Build history of the part. All positions in model axes, mm. A direction names the side the tool comes from. Give positions to 0.01 mm unless a question says otherwise; leave off trailing zeros. Loops run counter-clockwise (first coordinate to the right, second up) from the corner with the lowest first, then second, coordinate; pieces in that order, holes last. Notation, with made-up numbers: M 50.25,62.5 L 90.25,62.5 A18 cw 90.25,91.5 Z; hole C -35.5,85.25 d5. An arc over 180 degrees is marked long. Answer in a Markdown table with one row per item. Add a question column.
```python
from build123d import *

# Parameters (mm, degrees)
F1_DEPTH = 7.62
F2_DEPTH = 3.81


with BuildPart() as f1:
    # F0 (on Front) → F1 (new body)
    with BuildSketch(Plane.XZ):
        Polygon((0, 52.186977), (-15.490659, 28.424604), (-15.490659, -28.424604), (0, -52.487765), (15.490659, -28.424604), (15.490659, 28.424604), align=None)
        Polygon((-6.466974, -17.596183), (-6.466974, 17.596183), (0, 28.424604), (6.466974, 17.596183), (6.466974, -17.596183), (0, -28.424604), align=None, mode=Mode.SUBTRACT)
    extrude(amount=F1_DEPTH)

    # F0 (on Front) → F2 (join)
    with BuildSketch(Plane.XZ):
        Polygon((0, 28.424604), (-6.466974, 17.596183), (-6.466974, -17.596183), (0, -28.424604), (6.466974, -17.596183), (6.466974, 17.596183), align=None)
    extrude(amount=F2_DEPTH)


solid = f1.part
```
(1) Slice it at B-B, the plane z = -1.5. Give the cut face in (x, y), then the cut area to 3 significant figures.
(2) Slice it at C-C, the plane y = -2.5. Give the cut face in (x, z), then the cut area to 3 significant figures.
(3) Tool access for faces 5 (the flat face through (0, -3.81, 0)), 6 (the flat face through (-7.64, -3.76, 40.47)): list every direction of +Z, -Z, +X, -X, +Y, -Y with a clear straight run to the whole face (end or side of a thin tool).
(4) Slice it at A-A, the plane y = -6.5. Give the cut face in (x, z), then the cut area to 3 significant figures.
(5) Pin check, flat tips, straight feed: pin 1 (6.5 mm diameter, centred on x = 2.5, z = -7, fed in from -Y); pin 2 (3 mm diameter, centred on x = 0.5, y = -5, fed in from -Z). Stop position of each tip, or through.
(6) Wall check: line 1 (X direction, y = -4.5, z = -7); line 2 (Z direction, x = 4, y = -6.5); line 3 (Z direction, x = -3, y = -5.25). Give the ranges that are in metal, low to high.
(7) Pull direction X, two halves, no side cores. Call faces 1 (the flat face through (-15.491, -4, 0)), 2 (the flat face through (7.854, -3.757, 40.139)), 3 (the flat face through (3.188, -5.688, 23.086)), 4 (the flat face through (-3.3, -5.7, 22.9)): +X half, -X half, draft (parallel to the pull), parting line (faces both ways), or undercut.
(8) Slice it at D-D, the plane x = 12. Give the cut face in (y, z), then the cut area to 3 significant figures.
Solution:
| question | item | result |
|---|---|---|
| 1 | outline | M -15.49,-7.62 L -6.47,-7.62 L -6.47,-3.81 L 6.47,-3.81 L 6.47,-7.62 L 15.49,-7.62 L 15.49,0 L -15.49,0 Z |
| 1 | area | 187 mm^2 |
| 2 | outline | M -15.49,-28.42 L 0,-52.49 L 15.49,-28.42 L 15.49,28.42 L 0,52.19 L -15.49,28.42 Z |
| 2 | area | 2,500 mm^2 |
| 3 | face 5 | -Y |
| 3 | face 6 | +Z, -X, +Y, -Y |
| 4 | outline | M -15.49,-28.42 L 0,-52.49 L 15.49,-28.42 L 15.49,28.42 L 0,52.19 L -15.49,28.42 Z; hole M -6.47,-17.6 L 0,-28.42 L 6.47,-17.6 L 6.47,17.6 L 0,28.42 L -6.47,17.6 Z |
| 4 | area | 1,910 mm^2 |
| 5 | pin 1 | y = -3.81 |
| 5 | pin 2 | z = -52.49 |
| 6 | line 1 | -15.49 to -6.47, 6.47 to 15.49 |
| 6 | line 2 | -46.27 to -21.73, 21.73 to 46.05 |
| 6 | line 3 | -47.83 to -23.4, 23.4 to 47.59 |
| 7 | face 1 | -X half |
| 7 | face 2 | +X half |
| 7 | face 3 | undercut |
| 7 | face 4 | undercut |
| 8 | outline | M -7.62,-33.85 L 0,-33.85 L 0,33.78 L -7.62,33.78 Z |
| 8 | area | 515 mm^2 |
